```python
from build123d import *

# Parameters (mm, degrees)
F0_R           = 34.036
F0_R_2         = 6.35
F1_DEPTH       = 2.54
F2_R           = 12.7047221092
F3_DEPTH       = 25.4
F3_TAPER       = -15
F5_D           = 19.05
F5_CSINK_D     = 22.86
F5_CSINK_ANGLE = 90


with BuildPart() as f1:
    # F0 (on Top) → F1 (new body)
    with BuildSketch(Plane.XY):
        Circle(F0_R)
        Circle(F0_R_2, mode=Mode.SUBTRACT)
    extrude(amount=F1_DEPTH)

    # F2 (on Top) → F3 (join)
    with BuildSketch(Plane.XY):
        Circle(F2_R)
    extrude(amount=F3_DEPTH, taper=F3_TAPER)

    # F5 (through all)
    with Locations(Plane(origin=(0, 0, 0), x_dir=(1, 0, 0), z_dir=(0, 0, -1))):
        with Locations((0, 0)):
            CounterSinkHole(F5_D / 2, F5_CSINK_D / 2, counter_sink_angle=F5_CSINK_ANGLE)


solid = f1.part
```
Work out the finished part from the listing and answer in its coordinate system (mm). A direction names the side the tool comes from. Coordinates: 2 decimals unless noted, no trailing zeros. Write each loop counter-clockwise with the first axis right and the second up, starting at its lowest first coordinate (ties: lowest second). Pieces come first, ordered by that corner, then holes.
Q1. Determine the mould class of faces 1 (the face through (-12.006, -9.206, 9.05)), 2 (the face through (15, 0, 0)), 3 (the face through (7.559, 5.796, 13.817)) for opening direction Z: released by +Z, released by -Z, zero draft, split by the parting line, or undercut.
Q2. Which of the six approach directions +Z, -Z, +X, -X, +Y, -Y give full straight-line access (tool end or side, diameter ignored) to faces 4 (the face through (15, 0, 2.54)), 5 (the face through (-9, -4, 25.4))?
Q3. Find the intervals of material crossed by line 1 (Y direction, x = 0, z = 15.25) (3 decimals); line 2 (X direction, y = 2, z = 15.75); line 3 (Z direction, x = -12, y = -27.5), in increasing order.
Q4. A cutting plane is placed at C-C, the plane y = 29.5. Give the vertices of the cut face in (x, z).
Q5. Each of these flat-tipped pins is pushed along its axis until it touches: pin 1 Ø12 at (y, z) = (21, 17) entering from -X; pin 2 Ø4 at (x, y) = (4.5, 5) entering from +Z; pin 3 Ø3 at (y, z) = (-14.5, 9.5) entering from -X. Where does it stop, or does it pass through?
Q6. A cutting plane is placed at D-D, the plane z = 3.5. Give the vertices of the cut face in (x, y) (3 decimals).
Q7. A cutting plane is placed at A-A, the plane x = 0. Give the vertices of the cut face in (y, z) (3 decimals).
Q8. A cutting plane is placed at B-B, the plane z = 14.75. Give the vertices of the cut face in (x, y) (3 decimals), then the cut area to 3 significant figures.
Findings below:
1. face 1: undercut
1. face 2: released by -Z
1. face 3: zero draft
2. face 4: none
2. face 5: +Z, +X, -X, +Y, -Y
3. line 1: y = -16.791 to -9.525, 9.525 to 16.791
3. line 2: x = -16.81 to -9.31, 9.31 to 16.81
3. line 3: z = 0 to 2.54
4. outline: (-16.98, 0) - (16.98, 0) - (16.98, 2.54) - (-16.98, 2.54) - close
5. pin 1: stops at x = -9.02
5. pin 2: passes through
5. pin 3: stops at x = -8.09
6. outline: circle Ø27.285 at (0, 0); hole circle Ø19.05 at (0, 0)
7. outline: (-34.036, 0) - (-11.43, 0) - (-9.525, 1.905) - (-9.525, 25.4) - (-19.511, 25.4) - (-13.385, 2.54) - (-34.036, 2.54) - close; (9.525, 1.905) - (11.43, 0) - (34.036, 0) - (34.036, 2.54) - (13.385, 2.54) - (19.511, 25.4) - (9.525, 25.4) - close
8. outline: circle Ø33.314 at (0, 0); hole circle Ø19.05 at (0, 0)
8. area: 587 mm2
